Autodesk Inventor part; units mm, degrees
ref_plane "YZ Plane" through (0, 0, 0) normal (1, 0, 0) x (0, 1, 0)
ref_plane "XZ Plane" through (0, 0, 0) normal (0, 1, 0) x (-1, 0, 0)
ref_plane "XY Plane" through (0, 0, 0) normal (0, 0, 1) x (1, 0, 0)
sketch "Эскиз1" plane through (0, 0, 0) normal (0, 1, 0) x (-1, 0, 0)
  line L0 (7.1, -15.85) -> (-7.1, -15.85)
  line L1 (-7.1, -15.85) -> (-7.1, 15.85)
  line L2 (-7.1, 15.85) -> (7.1, 15.85)
  line L3 (7.1, 15.85) -> (7.1, -15.85)
  line L4 (7.1, -15.85) -> (-7.1, 15.85) construction
  line L5 (-7.1, -15.85) -> (7.1, 15.85) construction
  line L6 (9.1, -17.85) -> (-9.1, -17.85)
  line L7 (-9.1, -17.85) -> (-9.1, 17.85)
  line L8 (-9.1, 17.85) -> (9.1, 17.85)
  line L9 (9.1, 17.85) -> (9.1, -17.85)
  point P0 (0, 0)
  dimension "d0" = 14.2
  dimension "d1" = 31.7
  dimension "d2" = 2
extrude "Выдавливание1" add sketch "Эскиз1" along normal blind 10
sketch "Эскиз2" plane through (0, 10, 0) normal (0, 1, 0) x (1, 0, 0)
  line L0 (-9.1, 17.85) -> (-9.1, -17.85)
  line L1 (-9.1, -17.85) -> (9.1, -17.85)
  line L2 (9.1, -17.85) -> (9.1, 17.85)
  line L3 (9.1, 17.85) -> (-9.1, 17.85)
  point P0 (0, 0)
extrude "Выдавливание2" add sketch "Эскиз2" along normal blind 3
sketch "Эскиз4" plane through (9.1, 0, -17.85) normal (0, 0, -1) x (-1, 0, 0)
  line L0 (0, 0) -> (0, 13) construction
  line L1 (0, 0) -> (0, 13) construction
  line L2 (0, 0) -> (18.2, 0) construction
  line L3 (18.2, 0) -> (18.2, 13) construction
  line L4 (18.2, 0) -> (18.2, 13) construction
  line L5 (0, 0) -> (0, 13)
  line L6 (0, 0) -> (0, 13)
  line L7 (18.2, 0) -> (0, 0)
  line L8 (0, 0) -> (18.2, 0)
  line L9 (18.2, 0) -> (18.2, 13)
  line L10 (5.972, 13) -> (0, 13)
  line L11 (0, 13) -> (18.2, 13)
  line L12 (0, 0) -> (0, 13)
  line L13 (0, 13) -> (0, 7)
  line L14 (2, 0) -> (2, 10)
  line L15 (2, 10) -> (16.2, 10)
  line L16 (16.2, 10) -> (16.2, 0)
  point P0 (9.1, 0)
  point P1 (18.2, 7)
  point P2 (0, 6.5)
  point P3 (18.2, 6.5)
  point P4 (16.2, 0)
  dimension "d0" = 14.2
  dimension "d15" = 2
  dimension "d16" = 2
  dimension "d53" = 10
extrude "Выдавливание4" cut sketch "Эскиз4" against normal blind 3 contours L14 L15 L16 L7
sketch "Эскиз5" plane through (0, 13, 0) normal (0, 1, 0) x (1, 0, 0)
  line L0 (0, 0) -> (0, -28.4562) construction
  circle A0 centre (0, -22.85) radius 1.6
  circle A1 centre (0, 22.85) radius 1.6
  line L1 (-9.1, -17.85) -> (9.1, -17.85)
  line L2 (9.1, 17.85) -> (-9.1, 17.85)
  arc A2 (2.6208, 25.1698) -> (-2.6208, 25.1698) centre (0, 22.85) ccw
  arc A3 (-2.6208, -25.1698) -> (2.6208, -25.1698) centre (0, -22.85) ccw
  line L3 (9.1, 17.85) -> (-9.1, 17.85)
  line L4 (9.1, 17.85) -> (2.6208, 25.1698)
  line L5 (-9.1, 17.85) -> (-2.6208, 25.1698)
  line L6 (-9.1, -17.85) -> (-2.6208, -25.1698)
  line L7 (9.1, -17.85) -> (9.1, 17.85)
  line L8 (9.1, -17.85) -> (2.6208, -25.1698)
  point P0 (7.1, 17.85)
  dimension "d32" = 3.2
  dimension "d33" = 3.2
  dimension "d34" = 5
  dimension "d35" = 5
  dimension "d36" = 7
  dimension "d37" = 7
extrude "Выдавливание5" add sketch "Эскиз5" against normal blind 3
sketch "Эскиз6" plane through (0, 10, 0) normal (0, -1, 0) x (1, 0, 0)
  circle A0 centre (0, -8.65) radius 1.5 construction
  circle A1 centre (0, -8.65) radius 1.6
  point P0 (0, 0)
  dimension "d38" = 3.2
extrude "Выдавливание6" cut sketch "Эскиз6" against normal blind 10
chamfer "Фаска1" distance 1.65 angle 45 1 edges at (-1.6, 13, -8.65)
sketch "Эскиз7" plane through (0, 10, 0) normal (0, -1, 0) x (1, 0, 0)
  circle A0 centre (0, -8.65) radius 1.6
  circle A1 centre (0, -8.65) radius 1.6
  circle A2 centre (0, -8.65) radius 2.5
  point P0 (0, 0)
  dimension "d44" = 5
extrude "Выдавливание7" add sketch "Эскиз7" along normal blind 8.4
chamfer "Фаска3" distance 1 angle 45 1 edges at (-2.5, 10, -8.65)
properties part number "креп_опт" material "Полипропилен"
Read the model definition and answer for the solid it produces. Units are mm, in the model's axes. A direction names the side the tool comes from. Round coordinates to 2 decimals unless told otherwise and drop trailing zeros. Write each loop counter-clockwise with the first axis right and the second up, starting at its lowest first coordinate (ties: lowest second). Pieces come first, ordered by that corner, then holes. Notation, with made-up numbers: (24.5, 15.5) - (41.5, 15.5) arc R14 ccw to (41.5, 41.5) - close; hole circle Ø3 at (69.25, 19). An arc over 180 degrees is marked (long way). One line per question, with ' | ' between items. Start each with the question number.
1. Section D-D (y = 12) is taken. Determine the outline of the cut face in (x, z).
2. Each of these flat-tipped pins is pushed along its axis until it touches: pin 1 (3 mm diameter, centred on x = 0, z = 22.85, fed in from -Y); pin 2 (6 mm diameter, centred on x = 1.5, z = 5.5, fed in from -Y); pin 3 (1 mm diameter, centred on x = -3.5, y = 1.5, fed in from -Z); pin 4 (1.6 mm diameter, centred on x = 8.5, y = 5, fed in from -Z). Where does it stop, or does it pass through?
3. Section B-B (x = 0) is taken. Determine the outline of the cut face in (y, z).
4. Section C-C (z = -8.65) is taken. Determine the outline of the cut face in (x, y).
5. For a pull along X with two mould halves and no side action, classify faces 5 (the face through (5.906, 11.521, 21.459)), 6 (the face through (-5.906, 11.521, 21.459)), 7 (the face through (2, 1.6, -9)) as +X half, -X half, draft (parallel to the pull), parting line (faces both ways), or undercut.
6. Find the intervals of material crossed by probe 1 along Z at (x, y) = (0, 11.1); probe 2 along Z at (x, y) = (0, 12.25); probe 3 along X at (y, z) = (2.5, -8.5), in increasing order. Write a range as [from, to].
7. Section A-A (y = 3.5) is taken. Determine the outline of the cut face in (x, z).
8. For faces 1 (the face through (0, 5, 15.85)), 2 (the face through (-8, 5, -17.85)), 3 (the face through (-7.1, 5, -1)), 4 (the face through (0, 5, 17.85)), determine the directions among +Z, -Z, +X, -X, +Y, -Y from which every point of the face is accessible in a straight line to the end or side of a thin tool.
Filled in:
1) outline: (-9.1, -17.85) - (-2.62, -25.17) arc R3.5 ccw to (2.62, -25.17) - (9.1, -17.85) - (9.1, 17.85) - (2.62, 25.17) arc R3.5 ccw to (-2.62, 25.17) - (-9.1, 17.85) - close; hole circle Ø4.5 at (0, -8.65); hole circle Ø3.2 at (0, -22.85); hole circle Ø3.2 at (0, 22.85)
2) pin 1: through | pin 2: y = 10 | pin 3: z = 15.85 | pin 4: z = -17.85
3) outline: (0, 15.85) - (10, 15.85) - (10, -5.15) - (9, -6.15) - (1.6, -6.15) - (1.6, -7.05) - (11.35, -7.05) - (13, -5.4) - (13, 21.25) - (10, 21.25) - (10, 17.85) - (0, 17.85) - close; (1.6, -11.15) - (9, -11.15) - (10, -12.15) - (10, -21.25) - (13, -21.25) - (13, -11.9) - (11.35, -10.25) - (1.6, -10.25) - close; (10, -26.35) - (13, -26.35) - (13, -24.45) - (10, -24.45) - close; (10, 24.45) - (13, 24.45) - (13, 26.35) - (10, 26.35) - close
4) outline: (-9.1, 0) - (-7.1, 0) - (-7.1, 10) - (-3.5, 10) - (-2.5, 9) - (-2.5, 1.6) - (-1.6, 1.6) - (-1.6, 11.35) - (-3.25, 13) - (-9.1, 13) - close; (1.6, 1.6) - (2.5, 1.6) - (2.5, 9) - (3.5, 10) - (7.1, 10) - (7.1, 0) - (9.1, 0) - (9.1, 13) - (3.25, 13) - (1.6, 11.35) - close
5) face 5: +X half | face 6: -X half | face 7: undercut
6) probe 1: [-26.35, -24.45], [-21.25, -10.25], [-7.05, 21.25], [24.45, 26.35] | probe 2: [-26.35, -24.45], [-21.25, -11.15], [-6.15, 21.25], [24.45, 26.35] | probe 3: [-9.1, -7.1], [-2.5, -1.59], [1.59, 2.5], [7.1, 9.1]
7) outline: (-9.1, -17.85) - (-7.1, -17.85) - (-7.1, 15.85) - (7.1, 15.85) - (7.1, -17.85) - (9.1, -17.85) - (9.1, 17.85) - (-9.1, 17.85) - close; circle Ø5 at (0, -8.65); hole circle Ø3.2 at (0, -8.65)
8) face 1: -Y | face 2: -Z, +X, -X, -Y | face 3: -Z, -Y | face 4: +Z, +X, -X, -Y
